Model file for the job. Use its own axes, mm. A direction names the side the tool comes from. Round coordinates to 2 decimals unless told otherwise and drop trailing zeros. Write each loop counter-clockwise with the first axis right and the second up, starting at its lowest first coordinate (ties: lowest second). Pieces come first, ordered by that corner, then holes.
```python
from build123d import *

# Parameters (mm, degrees)
SKETCH3_W            = 42.5
SKETCH3_H            = 15
BOSS_EXTRUDE1_DEPTH  = 10
SKETCH2_R            = 7.012606221
CUT_EXTRUDE1_DEPTH   = 2.5
SKETCH11_W           = 42.5
SKETCH11_H           = 10
BOSS_EXTRUDE5_DEPTH  = 10
SKETCH14_W           = 42.5
SKETCH14_H           = 10
BOSS_EXTRUDE7_DEPTH  = 15
SKETCH20_W           = 10
SKETCH20_H           = 40
BOSS_EXTRUDE10_DEPTH = 50
SKETCH21_W           = 10
SKETCH21_H           = 25
BOSS_EXTRUDE11_DEPTH = 113.5
FILLET1_R            = 3
CHAMFER1_SIZE        = 15
CHAMFER1_SIZE2       = 30.41699103
FILLET2_R            = 3
CHAMFER2_SIZE        = 10
CHAMFER2_SIZE2       = 17.320508076
FILLET3_R            = 5
CUT_EXTRUDE2_DEPTH   = 144.583262507
FILLET4_R            = 3
FILLET5_R            = 1.5
SKETCH25_W           = 10
SKETCH25_H           = 14.5
BOSS_EXTRUDE12_DEPTH = 20
SKETCH26_W           = 20
SKETCH26_H           = 14.5
BOSS_EXTRUDE13_DEPTH = 10


with BuildPart() as part:
    # Sketch3 → Boss-Extrude1 (new body)
    with BuildSketch(Plane.XY):
        with Locations((-1.388845539, 0.05888455)):
            Rectangle(SKETCH3_W, SKETCH3_H)
    extrude(amount=-BOSS_EXTRUDE1_DEPTH)

    # Sketch2 → Cut-Extrude1 (cut)
    with BuildSketch(Plane.XY):
        Circle(SKETCH2_R)
        with BuildLine():
            Line((-16.888114198, 2.469689731), (-3.968626967, 4.5))
            ThreePointArc((-3.968626967, 4.5), (0, 6), (3.968626967, 4.5))
            Line((3.968626967, 4.5), (16.888114198, 2.469689731))
            ThreePointArc((16.888114198, 2.469689731), (19, 0), (16.888114198, -2.469689731))
            Line((16.888114198, -2.469689731), (3.968626967, -4.5))
            ThreePointArc((3.968626967, -4.5), (0, -6), (-3.968626967, -4.5))
            Line((-3.968626967, -4.5), (-16.888114198, -2.469689731))
            ThreePointArc((-16.888114198, -2.469689731), (-19, 0), (-16.888114198, 2.469689731))
        make_face()
    extrude(amount=-CUT_EXTRUDE1_DEPTH, mode=Mode.SUBTRACT)

    # Sketch11 → Boss-Extrude5 (add)
    with BuildSketch(Plane.XZ.offset(7.44111545)):
        with Locations((-1.388845539, -5)):
            Rectangle(SKETCH11_W, SKETCH11_H)
    extrude(amount=BOSS_EXTRUDE5_DEPTH)

    # Sketch14 → Boss-Extrude7 (add)
    with BuildSketch(Plane(origin=(0, 7.55888455, 0), x_dir=(1, 0, 0), z_dir=(0, 1, 0))):
        with Locations((-1.388845539, 5)):
            Rectangle(SKETCH14_W, SKETCH14_H)
    extrude(amount=BOSS_EXTRUDE7_DEPTH)

    # Sketch20 → Boss-Extrude10 (add)
    with BuildSketch(Plane.ZY.offset(22.638845539)):
        with Locations((-5, 2.55888455)):
            Rectangle(SKETCH20_W, SKETCH20_H)
    extrude(amount=BOSS_EXTRUDE10_DEPTH)

    # Sketch21 → Boss-Extrude11 (add)
    with BuildSketch(Plane.XY):
        with Locations((-60.138845539, 2.55888455)):
            Rectangle(SKETCH21_W, SKETCH21_H)
    extrude(amount=BOSS_EXTRUDE11_DEPTH)

    # Fillet1
    fillet1_edges = [part.edges().sort_by_distance(p)[0] for p in [
        (-65.138845539, 2.55888455, 0),
        (-60.138845539, -9.94111545, 0),
        (-55.138845539, 2.55888455, 0),
        (-60.138845539, 15.05888455, 0),
    ]]
    fillet(fillet1_edges, radius=FILLET1_R)

    # Chamfer1
    chamfer1_edges = [part.edges().sort_by_distance(p)[0] for p in [
        (19.861154461, 22.55888455, -5),
    ]]
    chamfer1_side = [part.faces().sort_by_distance(p)[0] for p in [
        (19.861154461, 2.55888455, -5),
    ]]
    chamfer(chamfer1_edges, length=CHAMFER1_SIZE, length2=CHAMFER1_SIZE2, reference=chamfer1_side[0])

    # Fillet2
    fillet2_edges = [part.edges().sort_by_distance(p)[0] for p in [
        (-10.555836569, 22.55888455, -5),
        (19.861154461, 7.55888455, -5),
    ]]
    fillet(fillet2_edges, radius=FILLET2_R)

    # Chamfer2
    chamfer2_edges = [part.edges().sort_by_distance(p)[0] for p in [
        (19.861154461, -17.44111545, -5),
    ]]
    chamfer2_side = [part.faces().sort_by_distance(p)[0] for p in [
        (19.861154461, -5.873875391, -5),
    ]]
    chamfer(chamfer2_edges, length=CHAMFER2_SIZE, length2=CHAMFER2_SIZE2, reference=chamfer2_side[0])

    # Fillet3
    fillet3_edges = [part.edges().sort_by_distance(p)[0] for p in [
        (2.540646385, -17.44111545, -5),
        (19.861154461, -7.44111545, -5),
    ]]
    fillet(fillet3_edges, radius=FILLET3_R)

    # Sketch24 → Cut-Extrude2 (cut, through all)
    with BuildSketch(Plane.ZY.offset(65.138845539)):
        Polygon((58.25, -6.94111545), (95.25, -6.94111545), (58.25, 12.05888455), (21.25, -6.94111545), align=None)
        Polygon((48.39896268, 12.05888455), (12.290027833, -6.483541453), (12.290027833, 12.05888455), align=None)
        Polygon((68.10103732, 12.05888455), (104.209972167, 12.05888455), (104.209972167, -6.483541453), align=None)
    extrude(amount=-CUT_EXTRUDE2_DEPTH, mode=Mode.SUBTRACT)

    # Fillet4
    fillet4_edges = [part.edges().sort_by_distance(p)[0] for p in [
        (-60.138845539, -6.483541453, 104.209972167),
        (-60.138845539, 12.05888455, 104.209972167),
        (-60.138845539, 12.05888455, 12.290027833),
        (-60.138845539, -6.483541453, 12.290027833),
        (-60.138845539, 12.05888455, 58.25),
    ]]
    fillet(fillet4_edges, radius=FILLET4_R)

    # Fillet5
    fillet5_edges = [part.edges().sort_by_distance(p)[0] for p in [
        (-60.138845539, 12.05888455, 68.10103732),
        (-60.138845539, 12.05888455, 48.39896268),
        (-60.138845539, -6.94111545, 21.25),
        (-60.138845539, -6.94111545, 95.25),
    ]]
    fillet(fillet5_edges, radius=FILLET5_R)

    # Sketch25 → Boss-Extrude12 (add)
    with BuildSketch(Plane.ZY.offset(72.638845539)):
        with Locations((-5, 2.55888455)):
            Rectangle(SKETCH25_W, SKETCH25_H)
    extrude(amount=BOSS_EXTRUDE12_DEPTH)

    # Sketch26 → Boss-Extrude13 (add)
    with BuildSketch(Plane.XY):
        with Locations((-82.638845539, 2.55888455)):
            Rectangle(SKETCH26_W, SKETCH26_H)
    extrude(amount=BOSS_EXTRUDE13_DEPTH)


solid = part.part
```
1) Which spindle directions (+Z, -Z, +X, -X, +Y, -Y) get a long thin tool onto all of the face, cutting with end or side? Do faces 4 (the face through (-83, 3, 10)), 5 (the face through (-72.639, 2, 5)), 6 (the face through (-54.24, 2.78, 0.86)), 7 (the face through (-60, 15.059, 57)), 8 (the face through (-60.07, 11.2, 13.19)). Say none if no direction does.
2) Pull direction X, two halves, no side cores. Call faces 1 (the face through (-83, -4.691, 0)), 2 (the face through (19.17, -7.09, -4.93)), 3 (the face through (0.09, 7.012, -1.232)): released by +X, released by -X, zero draft, split by the parting line, or undercut.
3) Cut at C-C on x = -23. List the corners of the cut face in (y, z).
4) Cut at A-A on z = 64. List the corners of the cut face in (x, y), and give its area (3 significant figures).
5) Flat gauge pins, fed straight in: pin 1 Ø5 at (x, z) = (-62.5, 77) entering from +Y; pin 2 Ø2 at (y, z) = (10, 96) entering from -X; pin 3 Ø3 at (x, z) = (-60.5, 30.5) entering from -Y; pin 4 Ø8 at (y, z) = (16.5, -6.5) entering from -X. Where does each tip first touch, or does it go through?
6) Cut at B-B on z = 35.5. List the corners of the cut face in (x, y), and give its area (3 significant figures).
7) Cut at D-D on x = -76. List the corners of the cut face in (y, z).
8) Wall check: probe 1 along X at (y, z) = (0.5, 5); probe 2 along X at (y, z) = (6.5, 104.5); probe 3 along Z at (x, y) = (-39.5, 6). Give the ranges that are in metal, low to high.
Result sheet:
1. face 4: +Z, -X, +Y, -Y
1. face 5: +Z, +Y, -Y
1. face 6: +Z, +X, +Y, -Y
1. face 7: +Z, +X, -X, +Y
1. face 8: +X, -X
2. face 1: zero draft
2. face 2: released by +X
2. face 3: undercut
3. outline: (-17.44, -10) - (22.56, -10) - (22.56, 0) - (-17.44, 0) - close
4. outline: (-65.14, -9.94) - (-55.14, -9.94) - (-55.14, -6.94) - (-65.14, -6.94) - close; (-65.14, 9.11) - (-55.14, 9.11) - (-55.14, 15.06) - (-65.14, 15.06) - close
4. area: 89.5 mm2
5. pin 1: stops at y = 15.06
5. pin 2: passes through
5. pin 3: stops at y = -9.94
5. pin 4: stops at x = -72.64
6. outline: (-65.14, -9.94) - (-55.14, -9.94) - (-55.14, -6.94) - (-65.14, -6.94) - close; (-65.14, 0.38) - (-55.14, 0.38) - (-55.14, 5.44) - (-65.14, 5.44) - close; (-65.14, 12.06) - (-55.14, 12.06) - (-55.14, 15.06) - (-65.14, 15.06) - close
6. area: 111 mm2
7. outline: (-4.69, -10) - (9.81, -10) - (9.81, 10) - (-4.69, 10) - close
8. probe 1: x = -92.64 to -72.64, -65.14 to -55.14
8. probe 2: x = -65.14 to -55.14
8. probe 3: z = -10 to 0
